Build history of the part. All positions in model axes, mm. A direction names the side the tool comes from. Give positions to 0.01 mm unless a question says otherwise; leave off trailing zeros. Write each loop counter-clockwise with the first axis right and the second up, starting at its lowest first coordinate (ties: lowest second). Pieces come first, ordered by that corner, then holes. Notation, with made-up numbers: (85, 10) -> (143, 10) arc R14 ccw to (143, 36) -> close; hole circle Ø11 at (2.5, -16.5). An arc over 180 degrees is marked (long way). One line per question, with ' | ' between items. Start each with the question number.
(1) Pin check, flat tips, straight feed: P1, Ø3, axis at x = 44, y = 3, coming from the +Z side; P2, Ø1.5, axis at x = 77, y = 3.5, coming from the -Z side. Stop position of each tip, or through.
(2) Tool access for faces 1 (the flat face through (160, 3, 0)), 2 (the flat face through (197, 3, -30)), 3 (the flat face through (6.35, 3, -40)), 4 (the flat face through (99, 0, -35)), 5 (the flat face through (150, 3, -72)): list every direction of +Z, -Z, +X, -X, +Y, -Y with a clear straight run to the whole face (end or side of a thin tool).
(3) Band-saw the part on A-A, the plane x = 166. Give the cut face in (y, z), and give its area (3 significant figures).
(4) Drill centre lines: probe 1 along X at (y, z) = (5, 0.5); probe 2 along X at (y, z) = (4.5, -40); probe 3 along Z at (x, y) = (31.5, 1.5). Where is each one in solid material? Low to high. Write a range as from..to.
from build123d import *

# Parameters (mm, degrees)
SKETCH1_W           = 30
SKETCH1_H           = 6.35
SKETCH1_W_2         = 20
BOSS_EXTRUDE1_DEPTH = 6.35


with BuildPart() as part:
    # Sketch1 → Boss-Extrude1 (new body)
    with BuildSketch(Plane(origin=(0, 0, 0), x_dir=(1, 0, 0), z_dir=(0, 1, 0))):
        Polygon((0, 30), (0, 0), (30, 0), (50, 0), (70, 0), (90, 0), (110, 0), (130, 0), (150, 0), (170, 0), (200, 0), (200, 30), (193.65, 30), (193.65, 50), (200, 50), (200, 75), (170, 75), (170, 68.65), (150, 68.65), (150, 75), (130, 75), (130, 68.65), (110, 68.65), (110, 75), (90, 75), (90, 68.65), (70, 68.65), (70, 75), (50, 75), (50, 68.65), (30, 68.65), (30, 75), (0, 75), (0, 50), (6.35, 50), (6.35, 30), align=None)
        with Locations((15, -3.175)):
            Rectangle(SKETCH1_W, SKETCH1_H)
        with Locations((60, -3.175)):
            Rectangle(SKETCH1_W_2, SKETCH1_H)
        with Locations((100, -3.175)):
            Rectangle(SKETCH1_W_2, SKETCH1_H)
        with Locations((140, -3.175)):
            Rectangle(SKETCH1_W_2, SKETCH1_H)
        with Locations((185, -3.175)):
            Rectangle(SKETCH1_W, SKETCH1_H)
    extrude(amount=BOSS_EXTRUDE1_DEPTH)


solid = part.part
Results:
1) P1: stops at z = 0 | P2: stops at z = -68.65
2) face 1: +Z, +Y, -Y | face 2: +X, +Y, -Y | face 3: -X, +Y, -Y | face 4: +Z, -Z, +X, -X, -Y | face 5: -Z, +Y, -Y
3) outline: (0, -68.65) -> (6.35, -68.65) -> (6.35, 0) -> (0, 0) -> close | area: 436 mm²
4) probe 1: x = 0..30, 50..70, 90..110, 130..150, 170..200 | probe 2: x = 6.35..193.65 | probe 3: z = -68.65..0
